The listing builds one solid part. Answer for the finished solid, in the listing's coordinates (mm). A direction names the side the tool comes from. Coordinates: 2 decimals unless noted, no trailing zeros. Loops run counter-clockwise (first coordinate to the right, second up) from the corner with the lowest first, then second, coordinate; pieces in that order, holes last. Notation, with made-up numbers: M 59,-16.75 L 86,-16.75 A14 cw 86,3.25 Z; hole C -26,-24 d10. An arc over 180 degrees is marked long. Answer as a JSON object with one key per item and string values. Group by question number.
1. A cutting plane is placed at A-A on y = 62. Give the vertices of the cut face in (x, z), and give its area (3 significant figures).
2. A cutting plane is placed at D-D on z = 16.5. Give the vertices of the cut face in (x, y).
3. Given pin 1 (1 mm diameter, centred on y = 59, z = 21, fed in from -X); pin 2 (4 mm diameter, centred on x = 9, z = 29, fed in from +Y); pin 3 (3 mm diameter, centred on y = 60.5, z = 28, fed in from -X); pin 4 (2 mm diameter, centred on x = 9.5, z = 26, fed in from -Y), each flat-ended and moving along its own axis, determine where each tip first touches the part or whether it passes through.
4. Straight lines are drawn through the part: L1, parallel to X at y = 63.25, z = 25; L2, parallel to X at y = 62.75, z = 4.5; L3, parallel to Y at x = 8.75, z = 6. For each, find the intervals that lie inside material, in ascending order.
5. For faces 1 (the face through (10.24, 63.983, 20.353)), 2 (the face through (10, 62, 36)), determine the directions among +Z, -Z, +X, -X, +Y, -Y from which every point of the face is accessible in a straight line to the end or side of a thin tool.
6. A cutting plane is placed at B-B on x = 10.5. Give the vertices of the cut face in (y, z).
7. A cutting plane is placed at C-C on z = 1.5. Give the vertices of the cut face in (x, y), and give its area (3 significant figures).
from build123d import *

# Parameters (mm, degrees)
CYLINDER007_R     = 2
CYLINDER007_DEPTH = 27


with BuildPart() as obj1:
    # Cylinder007 → Cylinder007 (new body)
    with BuildSketch(Plane(origin=(10.5, 62, 4), x_dir=(1, 0, 0), z_dir=(0, 0, 1))):
        Circle(CYLINDER007_R)
    extrude(amount=CYLINDER007_DEPTH)


with BuildPart() as kugel:
    # Sphere → Sphere (revolve)
    with BuildSketch(Plane(origin=(10.5, 62, -1), x_dir=(1, 0, 0), z_dir=(0, -1, 0))):
        with BuildLine():
            ThreePointArc((0, -4.15), (4.15, 0), (0, 4.15))
            Line((0, 4.15), (0, -4.15))
        make_face()
    revolve(axis=Axis((10.5, 62, -1), (0, 0, 1)))


with BuildPart() as kegel:
    # Cone → Cone (revolve)
    with BuildSketch(Plane(origin=(10.5, 62, 0), x_dir=(1, 0, 0), z_dir=(0, -1, 0))):
        Polygon((0, 0), (4, 0), (2, 10), (0, 10), align=None)
    revolve(axis=Axis((10.5, 62, 0), (0, 0, 1)))


with BuildPart() as fusion001:
    # Cone001 → Cone001 (revolve)
    with BuildSketch(Plane(origin=(10.5, 62, 31), x_dir=(1, 0, 0), z_dir=(0, -1, 0))):
        Polygon((0, 0), (2, 0), (1.8, 5), (0, 5), align=None)
    revolve(axis=Axis((10.5, 62, 31), (0, 0, 1)))

    # Fusion001: union obj1, Kugel, Kegel
    add(obj1.part)
    add(kugel.part)
    add(kegel.part)


solid = fusion001.part
From the geometry:
{
 "1": {"outline": "M 6.56,0.31 A4.15 ccw long 14.44,0.31 L 12.5,10 L 12.5,31 L 12.3,36 L 8.7,36 L 8.5,31 L 8.5,10 Z", "area": "198 mm²"},
 "2": {"outline": "C 10.5,62 d4"},
 "3": {"pin 1": "passes through", "pin 2": "stops at y = 64", "pin 3": "stops at x = 8.5", "pin 4": "stops at y = 60"},
 "4": {"L1": "x = 8.94 to 12.06", "L2": "x = 7.49 to 13.51", "L3": "y = 59.81 to 64.19"},
 "5": {"face 1": "+Z", "face 2": "+Z, +X, -X, +Y, -Y"},
 "6": {"outline": "M 58.06,0.31 A4.15 ccw long 65.94,0.31 L 64,10 L 64,31 L 63.8,36 L 60.2,36 L 60,31 L 60,10 Z"},
 "7": {"outline": "C 10.5,62 d7.4", "area": "43.0 mm²"}
}
